Job drawing, mm, ordinate dimensions from the low corner. One solid piece. A direction names the side the tool comes from. Coordinates: 2 decimals unless noted, no trailing zeros. Write each loop counter-clockwise with the first axis right and the second up, starting at its lowest first coordinate (ties: lowest second). Pieces come first, ordered by that corner, then holes. Notation, with made-up numbers: (76.25, 46) - (97.25, 46) arc R24 ccw to (97.25, 79) - close; hole circle Ø7 at (-30, -18.5). An arc over 180 degrees is marked (long way). Use a Markdown table: item, result.
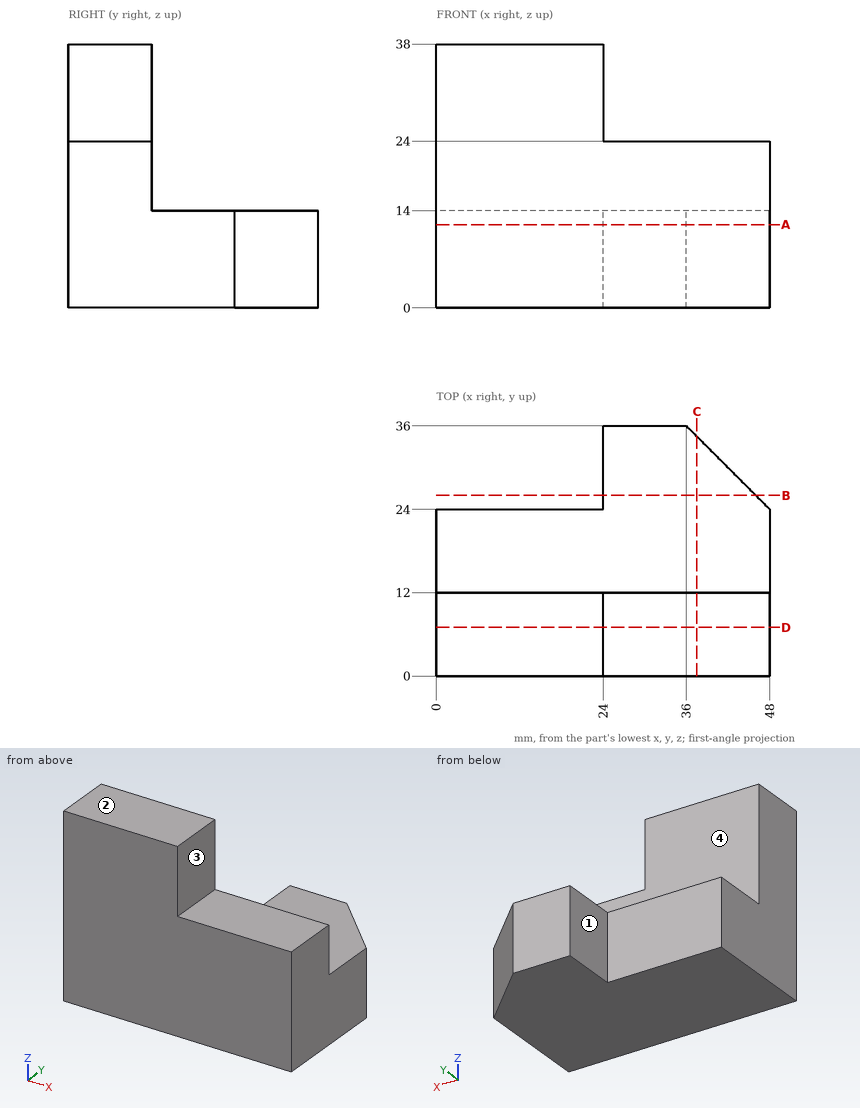
Item 1: Which spindle directions (+Z, -Z, +X, -X, +Y, -Y) get a long thin tool onto all of the face, cutting with end or side? Do the marked faces 1, 2, 3 and 4. Say none if no direction does.
From the geometry:
| item | result |
|---|---|
| face 1 | +Z, -Z, -X, +Y |
| face 2 | +Z, +X, -X, +Y, -Y |
| face 3 | +Z, +X, +Y, -Y |
| face 4 | +Z, +X, -X, +Y |
Item 2: Band-saw the part on B-B, the plane y = 26. Give the cut face in (x, z).
From the geometry:
| item | result |
|---|---|
| outline | (24, 0) - (46, 0) - (46, 14) - (24, 14) - close |
Item 3: Band-saw the part on A-A, the plane z = 12. Give the cut face in (x, y), then the cut area to 3 significant figures.
From the geometry:
| item | result |
|---|---|
| outline | (0, 0) - (48, 0) - (48, 24) - (36, 36) - (24, 36) - (24, 24) - (0, 24) - close |
| area | 1,370 mm^2 |
Item 4: Band-saw the part on D-D, the plane y = 7. Give the cut face in (x, z).
From the geometry:
| item | result |
|---|---|
| outline | (0, 0) - (48, 0) - (48, 24) - (24, 24) - (24, 38) - (0, 38) - close |
Item 5: Drill centre lines: probe 1 along Y at (x, z) = (8.5, 25); probe 2 along Y at (x, z) = (11.5, 8); probe 3 along Z at (x, y) = (33, 32.5). Where is each one in solid material? Low to high.
From the geometry:
| item | result |
|---|---|
| probe 1 | 0 to 12 |
| probe 2 | 0 to 24 |
| probe 3 | 0 to 14 |
Item 6: Drop flat-ended pins along their axis: P1, Ø13, axis at y = 7.5, z = 32.5, coming from the +X side; P2, Ø3, axis at x = 22, z = 11, coming from the +Y side; P3, Ø3.5, axis at y = 28, z = 6.5, coming from the -X side. Give the stop position or say it passes through.
From the geometry:
| item | result |
|---|---|
| P1 | x = 24 |
| P2 | y = 24 |
| P3 | x = 24 |
Item 7: Band-saw the part on C-C, the plane x = 37.5. Give the cut face in (y, z), then the cut area to 3 significant figures.
From the geometry:
| item | result |
|---|---|
| outline | (0, 0) - (34.5, 0) - (34.5, 14) - (12, 14) - (12, 24) - (0, 24) - close |
| area | 603 mm^2 |
